Could you check a few things on this model? Use its own coordinates, in mm. Face numbers are marked on the shaded views. Give positions to 0.01 mm unless a question says otherwise; leave off trailing zeros. Order: outer loops, then holes, each group sorted by start corner. A loop starts at its lowest first (then second) coordinate and runs counter-clockwise, first axis right, second up. Notation, with made-up numbers: (42, 42) -> (95, 42) arc R23 ccw to (95, 73) -> close; hole circle Ø4 at (-23.5, 15.25). An arc over 180 degrees is marked (long way). One line per item, written item: value.
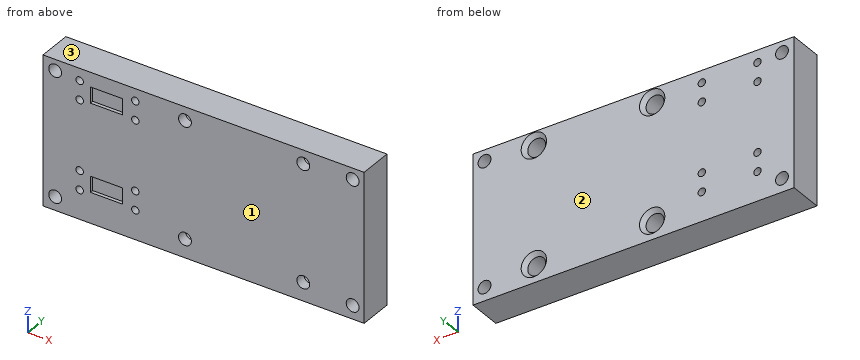
Autodesk Inventor part; units mm, degrees
ref_plane "YZ Plane" through (0, 0, 0) normal (1, 0, 0) x (0, 1, 0)
ref_plane "XZ Plane" through (0, 0, 0) normal (0, 1, 0) x (-1, 0, 0)
ref_plane "XY Plane" through (0, 0, 0) normal (0, 0, 1) x (1, 0, 0)
sketch "Sketch1" plane through (0, 0, 0) normal (0, 1, 0) x (-1, 0, 0)
  line L0 (46.6228, 34.6302) -> (-74.0272, 34.6302)
  line L1 (-74.0272, 34.6302) -> (-74.0272, -54.2698)
  line L2 (-74.0272, -54.2698) -> (46.6228, -54.2698)
  line L3 (46.6228, -54.2698) -> (46.6228, 34.6302)
  point P0 (0, 0)
  dimension "d0" = 120.65
  dimension "d1" = 88.9
extrude "Extrusion1" add sketch "Sketch1" along normal blind 12.7
sketch "Sketch2" plane through (0, 12.7, 0) normal (0, 1, 0) x (1, 0, 0)
  line L0 (-46.6228, -34.6302) -> (74.0272, -34.6302)
  line L1 (-46.6228, 54.2698) -> (-46.6228, -34.6302)
  point P0 (0, 0)
  point P1 (6.7172, -29.5502)
  point P2 (51.1672, -29.5502)
  dimension "d4" = 0
  dimension "d5" = 5.08
  dimension "d6" = 53.34
  dimension "d7" = 44.45
hole "Hole1" at (6.7172, 12.7, 29.5502) at (51.1672, 12.7, 29.5502) direction (0, -1, 0) diameter 4.826 depth 25.4 tip angle 118 countersink diameter 9.525 countersink angle 82
sketch "Sketch6" plane through (0, 0, 0) normal (0, -1, 0) x (1, 0, 0)
  line L0 (-46.6228, 34.6302) -> (74.0272, 34.6302)
  line L1 (-46.6228, -54.2698) -> (-46.6228, 34.6302)
  line L2 (74.0272, -54.2698) -> (-46.6228, -54.2698)
  point P0 (0, 0)
  point P1 (69.7092, -16.1698)
  point P2 (-42.0508, -16.1698)
  point P3 (-42.0508, 30.4392)
  point P4 (69.7092, 30.4392)
  dimension "d43" = 0
  dimension "d44" = 0
  dimension "d46" = 111.76
  dimension "d47" = 0
  dimension "d48" = 0
  dimension "d50" = 4.191
  dimension "d51" = 4.572
  dimension "d91" = 38.1
hole "Hole4" at (69.7092, 0, -16.1698) at (-42.0508, 0, -16.1698) at (-42.0508, 0, 30.4392) at (69.7092, 0, 30.4392) direction (0, 1, 0) diameter 4.8 depth 25.4 tip angle 118
sketch "Sketch10" plane through (0, 12.7, 0) normal (0, 1, 0) x (1, 0, 0)
  circle A0 centre (51.1672, -29.5502) radius 2.413
  circle A1 centre (6.7172, -29.5502) radius 2.413
  line L0 (74.0272, 54.2698) -> (-46.6228, 54.2698)
  point P0 (0, 0)
  point P1 (6.7172, 14.2648)
  point P2 (51.1672, 14.2648)
  point P3 (66.6772, 28.8698)
  point P4 (-45.6228, 28.8698)
  point P5 (-46.6228, 54.2698)
  dimension "d80" = 0
  dimension "d81" = 0
  dimension "d82" = 0
  dimension "d144" = 43.815
hole "Hole7" at (6.7172, 12.7, -14.2648) at (51.1672, 12.7, -14.2648) direction (0, -1, 0) diameter 4.826 end through all countersink diameter 9.525 countersink angle 82
sketch "Sketch11" plane through (0, 0, 0) normal (0, -1, 0) x (1, 0, 0)
  line L0 (-28.8428, 29.2002) -> (-16.8428, 29.2002)
  line L1 (-16.8428, 29.2002) -> (-16.8428, 23.2002)
  line L2 (-16.8428, 23.2002) -> (-28.8428, 23.2002)
  line L3 (-28.8428, 23.2002) -> (-28.8428, 29.2002)
  line L4 (-28.8428, -3.8198) -> (-16.8428, -3.8198)
  line L5 (-16.8428, -3.8198) -> (-16.8428, -9.8198)
  line L6 (-16.8428, -9.8198) -> (-28.8428, -9.8198)
  line L7 (-28.8428, -9.8198) -> (-28.8428, -3.8198)
  line L8 (-28.8428, 23.5502) -> (-28.8428, 29.5502)
  line L9 (-16.8428, 29.5502) -> (-16.8428, 23.5502)
  line L10 (74.0272, -54.2698) -> (-46.6228, -54.2698)
  point P0 (0, 0)
  dimension "d93" = 0
  dimension "d94" = 0
  dimension "d95" = 0
  dimension "d96" = 0
  dimension "d97" = 6
  dimension "d98" = 6
  dimension "d99" = 44.45
  dimension "d100" = 77.47
extrude "Extrusion4" cut sketch "Sketch11" against normal blind 1.27
sketch "Sketch12" plane through (0, 0, 0) normal (0, -1, 0) x (1, 0, 0)
  circle A0 centre (-42.0508, 30.4392) radius 2.4
  circle A1 centre (69.7092, 30.4392) radius 2.4
  circle A2 centre (69.7092, -16.1698) radius 2.4
  circle A3 centre (-42.0508, -16.1698) radius 2.4
  point P0 (0, 0)
hole "Hole8" at (-42.0508, 0, 30.4392) at (69.7092, 0, 30.4392) at (69.7092, 0, -16.1698) at (-42.0508, 0, -16.1698) direction (0, 1, 0) diameter 4.826 end through all
sketch "Sketch13" plane through (0, 0, 0) normal (0, -1, 0) x (1, 0, 0)
  circle A0 centre (-32.8428, -42.0898) radius 1.4
  circle A1 centre (-32.8428, -49.1898) radius 1.4
  line L0 (-46.6228, 34.6302) -> (74.0272, 34.6302)
  circle A2 centre (-11.9428, -42.0898) radius 1.4
  point P0 (0, 0)
  point P1 (-32.8428, -10.3398)
  point P2 (-32.8428, -3.2278)
  point P3 (-32.8428, 22.9462)
  point P4 (-32.8428, 30.0582)
  point P5 (-39.7887, 34.6302)
  point P6 (67.4471, 34.6302)
  point P7 (-11.9428, -10.3398)
  point P8 (-11.9428, -3.2278)
  point P9 (-11.9428, 22.9462)
  point P10 (-11.9428, 30.0582)
  dimension "d110" = 0
  dimension "d111" = 0
  dimension "d112" = 0
  dimension "d113" = 7.112
  dimension "d114" = 7.112
  dimension "d115" = 31.75
  dimension "d116" = 4.572
  dimension "d117" = 0
  dimension "d118" = 0
  dimension "d119" = 0
  dimension "d120" = 0
  dimension "d121" = 0
  dimension "d122" = 0
  dimension "d123" = 0
  dimension "d124" = 0
hole "Hole9" at (-32.8428, 0, -10.3398) at (-32.8428, 0, -3.2278) at (-32.8428, 0, 22.9462) at (-32.8428, 0, 30.0582) at (-11.9428, 0, -10.3398) at (-11.9428, 0, -3.2278) at (-11.9428, 0, 22.9462) at (-11.9428, 0, 30.0582) direction (0, 1, 0) diameter 2.8 end through all
sketch "Sketch15" plane through (0, 12.7, 0) normal (0, 1, 0) x (1, 0, 0)
  circle A0 centre (6.7172, 14.2648) radius 2.413
  circle A1 centre (51.1672, 14.2648) radius 2.413
  circle A2 centre (6.7172, -29.5502) radius 2.413
  circle A3 centre (51.1672, -29.5502) radius 2.413
  circle A4 centre (6.7172, 14.2648) radius 3.3734
  circle A5 centre (6.7172, -29.5502) radius 3.3734
  circle A6 centre (51.1672, -29.5502) radius 3.3734
  circle A7 centre (51.1672, 14.2648) radius 3.3734
  point P0 (0, 0)
  dimension "d138" = 6.7469
  dimension "d139" = 6.7469
  dimension "d140" = 6.7469
  dimension "d141" = 6.7469
extrude "Extrusion6" cut sketch "Sketch15" against normal blind 8.89
sketch "Sketch16" plane through (0, 0, 0) normal (0, -1, 0) x (1, 0, 0)
  line L0 (-64.483, -21.2498) -> (91.0848, -21.2498)
  line L1 (91.0848, -21.2498) -> (91.0848, -72.9236)
  line L2 (91.0848, -72.9236) -> (-64.483, -72.9236)
  line L3 (-64.483, -72.9236) -> (-64.483, -21.2498)
  line L4 (74.0272, -54.2698) -> (-46.6228, -54.2698)
  point P0 (0, 0)
  dimension "d145" = 33.02
extrude "Extrusion7" cut sketch "Sketch16" against normal blind 25.4
equation "\"d52\" = LegoMainHole"
equation "\"d125\" = CanConHoleDiam"
equation "\"LegoMainHole\" = 4.8"
equation "\"TalonSRXWidth\" = 31.75"
equation "\"TalonSRXFromSide\" = 15.875"
equation "\"TalonSRXBetweenHoles\" = 50.8"
equation "\"CanConPinWidth\" = 6"
equation "\"CanConPinLength\" = 12"
equation "\"CanConBetweenSideHoles\" = 20.9"
equation "\"CanConBetweenTopHoles\" = 7.1"
equation "\"CanConHoleDiam\" = 2.8"
equation "\"CanConHoleFromTopPin\" = 4"
properties part number "OneSparkMaxPlate"
1) Suppose I cut it at B-B, the plane x = -26.5. Write out the boundary of the cut face in (y, z).
Answer below:
outline: (0, -21.25) -> (12.7, -21.25) -> (12.7, 34.63) -> (0, 34.63) -> (0, 29.2) -> (1.27, 29.2) -> (1.27, 23.2) -> (0, 23.2) -> (0, -3.82) -> (1.27, -3.82) -> (1.27, -9.82) -> (0, -9.82) -> close
2) We'd pull the mould along Y, two halves only. Please class the marked faces 1, 2 and 3: +Y half, -Y half, draft (parallel to the pull), parting line (faces both ways), or undercut.
Answer below:
face 1: -Y half
face 2: +Y half
face 3: draft
3) For P1, Ø5.5, axis at x = 6.72, z = -14.26, coming from the +Y side; P2, Ø1.8, axis at x = -25.5, z = -6.5, coming from the -Y side; P3, Ø2, axis at x = -32.84, z = 30.06, coming from the -Y side; P4, Ø7.5, axis at x = 52, z = -14.5, coming from the +Y side, each with a flat end and sliding along its axis, tell me the tip position at first contact or that it passes through.
Answer below:
P1: stops at y = 3.81
P2: stops at y = 1.27
P3: passes through
P4: stops at y = 12.53
4) If I drill on line 1 along Z through (x, y) = (-24.5, 1); line 2 along Z through (x, y) = (6, 6); line 3 along X through (y, z) = (11.25, -12), over which ranges is the centre line in solid material (lowest first)?
Answer below:
line 1: z = -21.25 to -9.82, -3.82 to 23.2, 29.2 to 34.63
line 2: z = -21.25 to -17.56, -10.97 to 26.25, 32.85 to 34.63
line 3: x = -46.62 to 4.05, 9.39 to 48.5, 53.84 to 74.03
5) Suppose I cut it at A-A, the plane y = 9. State how many separate pieces and enclosed holes the cut face has, then the cut area to 3 significant figures.
Answer below:
separate pieces: 1
enclosed holes: 16
area: 6,480 mm2
